Part model, mm, in its own coordinate system. Give positions to 0.01 mm unless a question says otherwise; leave off trailing zeros. Order: outer loops, then holes, each group sorted by start corner. A loop starts at its lowest first (then second) coordinate and runs counter-clockwise, first axis right, second up. Notation, with made-up numbers: M 66.25,81 L 120.25,81 A24 ccw 120.25,117 Z; hole C -27.75,34 d7. An arc over 180 degrees is marked long. Answer as a JSON object with one key per item and string values.
from build123d import *

# Parameters (mm, degrees)
SKETCH1_W                                        = 635
SKETCH1_H                                        = 101.6
BOSS_EXTRUDE1_DEPTH                              = 12.7
F_33_64_0_51563_DIAMETER_HOLE1_D                 = 13.097002
CHAMFER1_SIZE                                    = 25.4
F_3_8_16_TAPPED_HOLE1_D                          = 7.9375
F_3_8_16_TAPPED_HOLE2_D                          = 7.9375
LPATTERN1_COUNT                                  = 2
LPATTERN1_PITCH                                  = 254
LPATTERN1_COUNT_DIR2                             = 2
LPATTERN1_PITCH_DIR2                             = 76.2
CBORE_FOR_3_8_SOCKET_HEAD_CAP_SCREW2_D           = 9.8044
CBORE_FOR_3_8_SOCKET_HEAD_CAP_SCREW2_CBORE_D     = 15.875
CBORE_FOR_3_8_SOCKET_HEAD_CAP_SCREW2_CBORE_DEPTH = 9.525


with BuildPart() as part:
    # Sketch1 → Boss-Extrude1 (new body)
    with BuildSketch(Plane(origin=(0, 0, 0), x_dir=(0, 0, -1), z_dir=(1, 0, 0))):
        with Locations((317.5, 50.8)):
            Rectangle(SKETCH1_W, SKETCH1_H)
    extrude(amount=BOSS_EXTRUDE1_DEPTH)

    # 33/64 (0.51563) Diameter Hole1 (through all)
    with Locations(Plane(origin=(12.7, 0, 0), x_dir=(0, 0, -1), z_dir=(1, 0, 0))):
        with Locations((38.1, 50.8), (596.9, 50.8)):
            Hole(F_33_64_0_51563_DIAMETER_HOLE1_D / 2)

    # Chamfer1
    chamfer1_edges = [part.edges().sort_by_distance(p)[0] for p in [
        (6.35, 101.6, 0),
        (6.35, 101.6, -635),
        (6.35, 0, -635),
        (6.35, 0, 0),
    ]]
    chamfer(chamfer1_edges, length=CHAMFER1_SIZE)

    # 3/8-16 Tapped Hole1 (through all)
    with Locations(Plane.ZY):
        with Locations((-622.3, 25.4), (-571.5, 25.4), (-63.5, 25.4), (-12.7, 25.4)):
            Hole(F_3_8_16_TAPPED_HOLE1_D / 2)

    # 3/8-16 Tapped Hole2 (through all)
    with Locations(Plane(origin=(12.7, 0, 0), x_dir=(0, 0, -1), z_dir=(1, 0, 0))):
        with Locations((190.5, 12.7)):
            f_3_8_16_tapped_hole2 = Hole(F_3_8_16_TAPPED_HOLE2_D / 2)

    # LPattern1: 3_8-16 Tapped Hole2 2 × 2
    with Locations(*[(0, j * LPATTERN1_PITCH_DIR2, -i * LPATTERN1_PITCH) for i in range(LPATTERN1_COUNT) for j in range(LPATTERN1_COUNT_DIR2) if (i, j) != (0, 0)]):
        add(f_3_8_16_tapped_hole2, mode=Mode.SUBTRACT)

    # CBORE for 3/8 Socket Head Cap Screw2 (through all)
    with Locations(Plane(origin=(12.7, 0, 0), x_dir=(0, 0, -1), z_dir=(1, 0, 0))):
        with Locations((241.3, 50.8), (393.7, 50.8)):
            CounterBoreHole(CBORE_FOR_3_8_SOCKET_HEAD_CAP_SCREW2_D / 2, CBORE_FOR_3_8_SOCKET_HEAD_CAP_SCREW2_CBORE_D / 2, CBORE_FOR_3_8_SOCKET_HEAD_CAP_SCREW2_CBORE_DEPTH)


solid = part.part
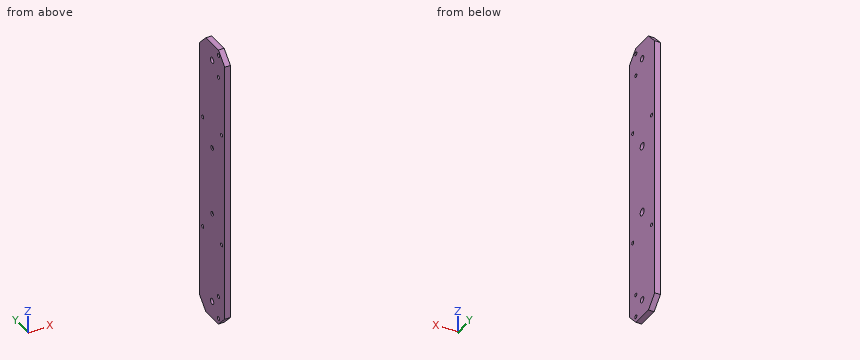
1. Cut at A-A on z = -596.9. Give the cut face in (x, y), plus the area to 3 significant figures.
Worked answers:
{"outline": "M 0,0 L 12.7,0 L 12.7,44.25 L 0,44.25 Z; M 0,57.35 L 12.7,57.35 L 12.7,101.6 L 0,101.6 Z", "area": "1,120 mm^2"}
2. Pin check, flat tips, straight feed: P1, Ø12.5, axis at y = 49.5, z = -241, coming from the +X side (3 decimals); P2, Ø10.5, axis at y = 50.8, z = -596.9, coming from the -X side. Stop position of each tip, or through.
Worked answers:
{"P1": "stops at x = 3.175", "P2": "passes through"}
3. Cut at B-B on x = 5.5. State how many separate pieces and enclosed holes the cut face has, plus the area to 3 significant figures.
Worked answers:
{"separate pieces": "1", "enclosed holes": "12", "area": "62,200 mm^2"}
4. Probe line 1 along Y through (x, z) = (5.25, -190.5); line 2 along Y through (x, z) = (9.75, -241.3); line 3 along Z through (x, y) = (9.25, 89). List the from-to ranges inside material, lowest first.
Worked answers:
{"line 1": "y = 0 to 8.73, 16.67 to 84.93, 92.87 to 101.6", "line 2": "y = 0 to 42.86, 58.74 to 101.6", "line 3": "z = -622.2 to -448.47, -440.53 to -194.47, -186.53 to -12.8"}
